from build123d import *

# Parameters (mm, degrees)
EXTRUDE_1_DEPTH     = 41
FILLET_1_R          = 12
SKETCH_2_R          = 5
CUT_EXTRUDE_1_DEPTH = 82


with BuildPart() as part:
    # 草圖1 → 伸長1 (new, symmetric)
    with BuildSketch(Plane.XY):
        Polygon((-30, 0), (30, 0), (30, 4), (68, 4), (68, 16), (24, 16), (24, 12), (-24, 12), (-24, 16), (-68, 16), (-68, 4), (-30, 4), align=None)
    extrude(amount=EXTRUDE_1_DEPTH, both=True)

    # 圓角1
    fillet_1_edges = [part.edges().sort_by_distance(p)[0] for p in [
        (68, 10, 41),
        (-68, 10, -41),
        (68, 10, -41),
        (-68, 10, 41),
    ]]
    fillet(fillet_1_edges, radius=FILLET_1_R)

    # 草圖2 → 除料-伸長1 (cut, through all)
    with BuildSketch(Plane(origin=(0, 16, 0), x_dir=(-1, 0, 0), z_dir=(0, 1, 0))):
        with Locations((-56, -29)):
            Circle(SKETCH_2_R)
        with Locations((-56, 29)):
            Circle(SKETCH_2_R)
        with Locations((56, -29)):
            Circle(SKETCH_2_R)
        with Locations((56, 29)):
            Circle(SKETCH_2_R)
    extrude(amount=-CUT_EXTRUDE_1_DEPTH, mode=Mode.SUBTRACT)


solid = part.part
Design review of the part built by this model. Coordinates are the model's own, in mm. A direction names the side the tool comes from. Coordinates: 2 decimals unless noted, no trailing zeros. Write each loop counter-clockwise with the first axis right and the second up, starting at its lowest first coordinate (ties: lowest second). Pieces come first, ordered by that corner, then holes. Notation, with made-up numbers: (-12.5, 43.25) -> (46.5, 43.25) arc R26 ccw to (46.5, 76.25) -> close; hole circle Ø2 at (20.25, 51). An arc over 180 degrees is marked (long way). Write each question's results on one line, items separated by ' | '. Start each with the question number.
(1) Take a section at B-B on y = 8.75. Write out the cut boundary in (x, z).
(2) The part is to be moulded in two halves that separate along Z. For faces 4 (the face through (-52, 10, -32)), 5 (the face through (-49, 4, 1)), 6 (the face through (-1, 8, 41)), 7 (the face through (60, 10, -32)), say which applies: pulls with the +Z half, pulls with the -Z half, needs draft (parallel to the pull), parting line crosses it, or undercut.
(3) For line 1 along Z through (x, y) = (-56, 12.25); line 2 along X through (y, z) = (5.5, -31.5); line 3 along Z through (x, y) = (-54.5, 8.25), list the stretches that pass through material, from the lowest coordinate up. Write a range as from..to.
(4) Take a section at A-A on z = 2. Write out the cut boundary in (x, y).
(5) Tool access review of faces 1 (the face through (0, 12, 1)), 2 (the face through (49, 4, 1)), 3 (the face through (-30, 2, 1)): name each direction out of +Z, -Z, +X, -X, +Y, -Y from which nothing blocks a thin tool from reaching the whole face with its end or side.
(6) Take a section at C-C on x = -58. Write out the cut boundary in (y, z), and give its area (3 significant figures).
(7) Clearance check with flat-ended pins moving along their axes: P1, Ø2, axis at y = 2, z = -10, coming from the -X side; P2, Ø13, axis at x = 56, z = 29, coming from the +Y side; P3, Ø24, axis at x = -7, z = -7, coming from the +Y side; P4, Ø11.5, axis at x = 54, z = 0, coming from the -Y side. State where each tip first meets the part, or that it passes through.
(8) Take a section at D-D on x = 32.5. Write out the cut boundary in (y, z).
Results found:
1) outline: (-68, -29) arc R12 ccw to (-56, -41) -> (56, -41) arc R12 ccw to (68, -29) -> (68, 29) arc R12 ccw to (56, 41) -> (-56, 41) arc R12 ccw to (-68, 29) -> close; hole circle Ø10 at (-56, -29); hole circle Ø10 at (-56, 29); hole circle Ø10 at (56, -29); hole circle Ø10 at (56, 29)
2) face 4: undercut | face 5: needs draft | face 6: pulls with the +Z half | face 7: undercut
3) line 1: z = -41..-34, -24..24, 34..41 | line 2: x = -67.74..-60.33, -51.67..51.67, 60.33..67.74 | line 3: z = -41..-33.77, -24.23..24.23, 33.77..41
4) outline: (-68, 4) -> (-30, 4) -> (-30, 0) -> (30, 0) -> (30, 4) -> (68, 4) -> (68, 16) -> (24, 16) -> (24, 12) -> (-24, 12) -> (-24, 16) -> (-68, 16) -> close
5) face 1: +Z, -Z, +Y | face 2: +Z, -Z, +X, -Y | face 3: +Z, -Z, -X, -Y
6) outline: (4, -40.83) -> (16, -40.83) -> (16, -33.58) -> (4, -33.58) -> close; (4, -24.42) -> (16, -24.42) -> (16, 24.42) -> (4, 24.42) -> close; (4, 33.58) -> (16, 33.58) -> (16, 40.83) -> (4, 40.83) -> close | area: 760 mm2
7) P1: stops at x = -30 | P2: stops at y = 16 | P3: stops at y = 12 | P4: stops at y = 4
8) outline: (4, -41) -> (16, -41) -> (16, 41) -> (4, 41) -> close
